The listing builds one solid part. Answer for the finished solid, in the listing's coordinates (mm). Face numbers are marked on the shaded views. A direction names the side the tool comes from. Round coordinates to 2 decimals unless told otherwise and drop trailing zeros. Write each loop counter-clockwise with the first axis right and the second up, starting at its lowest first coordinate (ties: lowest second). Pieces come first, ordered by that corner, then holes.
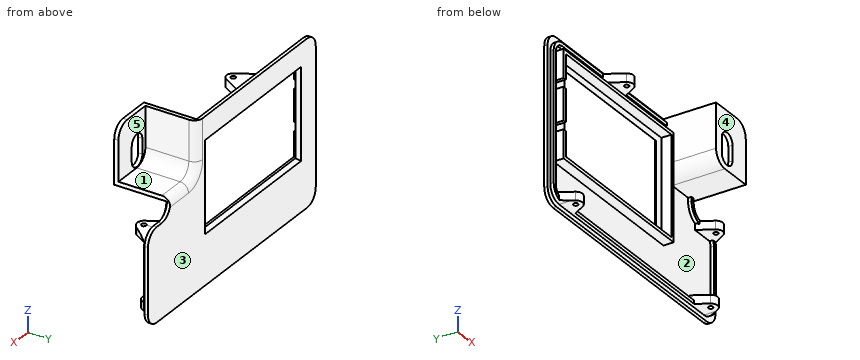
from build123d import *

# Parameters (mm, degrees)
BOSS_EXTRUDE1_DEPTH = 2
BOSS_EXTRUDE2_DEPTH = 2
SKETCH3_W           = 27.22
SKETCH3_H           = 33.28
BOSS_EXTRUDE3_DEPTH = 2.5
SKETCH4_W           = 31.75
SKETCH4_H           = 33.28
BOSS_EXTRUDE4_DEPTH = 2.5
SKETCH5_W           = 27.22
SKETCH5_H           = 34.25
BOSS_EXTRUDE5_DEPTH = 2.5
FILLET1_R           = 8
CUT_EXTRUDE1_REACH  = 98.066
FILLET3_R           = 8
FILLET6_R           = 5
SKETCH7_W           = 101
SKETCH7_H           = 62.8
SKETCH7_W_2         = 97
SKETCH7_H_2         = 58.8
BOSS_EXTRUDE6_DEPTH = 6
CUT_EXTRUDE2_REACH  = 98.896
SKETCH8_W           = 84
SKETCH8_H           = 50
CHAMFER1_SIZE       = 2
BOSS_EXTRUDE7_START = -2.5
SKETCH9_R           = 1.4
BOSS_EXTRUDE7_DEPTH = 5
BOSS_EXTRUDE8_START = 3.75
SKETCH10_R          = 1.4
BOSS_EXTRUDE8_DEPTH = 5
SKETCH11_R          = 1.4
BOSS_EXTRUDE9_DEPTH = 5
CUT_EXTRUDE3_DEPTH  = 97.22727472
SKETCH13_W          = 2
SKETCH13_H          = 5
CUT_EXTRUDE4_DEPTH  = 6


with BuildPart() as part:
    # Sketch1 → Boss-Extrude1 (new body)
    with BuildSketch(Plane(origin=(0, 0, 0), x_dir=(1, 0, 0), z_dir=(0, 1, 0))):
        with BuildLine():
            Line((-77, 40.5), (-77, -40.5))
            ThreePointArc((-77, -40.5), (-74.656854249, -46.156854249), (-69, -48.5))
            Line((-69, -48.5), (29.28, -48.5))
            Line((29.28, -48.5), (29.28, -46))
            Line((29.28, -46), (29.28, -14.25))
            Line((29.28, -14.25), (54, -14.25))
            Line((54, -14.25), (56.5, -14.25))
            ThreePointArc((56.5, -14.25), (58.843145751, -8.593145751), (64.5, -6.25))
            Line((64.5, -6.25), (69, -6.25))
            ThreePointArc((69, -6.25), (74.656854249, -3.906854249), (77, 1.75))
            Line((77, 1.75), (77, 40.5))
            ThreePointArc((77, 40.5), (74.656854249, 46.156854249), (69, 48.5))
            Line((69, 48.5), (-69, 48.5))
            ThreePointArc((-69, 48.5), (-74.656854249, 46.156854249), (-77, 40.5))
        make_face()
    extrude(amount=BOSS_EXTRUDE1_DEPTH)

    # Sketch2 → Boss-Extrude2 (add)
    with BuildSketch(Plane.XZ):
        with BuildLine():
            Line((54, 11.75), (54, 14.25))
            Line((54, 14.25), (52, 14.25))
            Line((52, 14.25), (52, 11.75))
            ThreePointArc((52, 11.75), (54.928932188, 4.678932188), (62, 1.75))
            Line((62, 1.75), (66.5, 1.75))
            ThreePointArc((66.5, 1.75), (70.742640687, -0.007359313), (72.5, -4.25))
            Line((72.5, -4.25), (72.5, -38))
            ThreePointArc((72.5, -38), (70.742640687, -42.242640687), (66.5, -44))
            Line((66.5, -44), (-66.5, -44))
            ThreePointArc((-66.5, -44), (-70.742640687, -42.242640687), (-72.5, -38))
            Line((-72.5, -38), (-72.5, 38))
            ThreePointArc((-72.5, 38), (-70.742640687, 42.242640687), (-66.5, 44))
            Line((-66.5, 44), (29.28, 44))
            Line((29.28, 44), (29.28, 46))
            Line((29.28, 46), (-66.5, 46))
            ThreePointArc((-66.5, 46), (-72.156854249, 43.656854249), (-74.5, 38))
            Line((-74.5, 38), (-74.5, -38))
            ThreePointArc((-74.5, -38), (-72.156854249, -43.656854249), (-66.5, -46))
            Line((-66.5, -46), (66.5, -46))
            ThreePointArc((66.5, -46), (72.156854249, -43.656854249), (74.5, -38))
            Line((74.5, -38), (74.5, -4.25))
            ThreePointArc((74.5, -4.25), (72.156854249, 1.406854249), (66.5, 3.75))
            Line((66.5, 3.75), (62, 3.75))
            ThreePointArc((62, 3.75), (56.343145751, 6.093145751), (54, 11.75))
        make_face()
    extrude(amount=BOSS_EXTRUDE2_DEPTH)

    # Sketch3 → Boss-Extrude3 (add)
    with BuildSketch(Plane.XY.offset(14.25)):
        with Locations((42.89, -14.64)):
            Rectangle(SKETCH3_W, SKETCH3_H)
    extrude(amount=BOSS_EXTRUDE3_DEPTH)

    # Sketch4 → Boss-Extrude4 (add)
    with BuildSketch(Plane(origin=(29.28, 0, 0), x_dir=(0, 0, -1), z_dir=(1, 0, 0))):
        with Locations((-32.625, -14.64)):
            Rectangle(SKETCH4_W, SKETCH4_H)
    extrude(amount=BOSS_EXTRUDE4_DEPTH)

    # Sketch5 → Boss-Extrude5 (add)
    with BuildSketch(Plane.XZ.offset(31.28)):
        with Locations((42.89, 31.375)):
            Rectangle(SKETCH5_W, SKETCH5_H)
    extrude(amount=-BOSS_EXTRUDE5_DEPTH)

    # Fillet1
    fillet1_edges = [part.edges().sort_by_distance(p)[0] for p in [
        (56.5, -30.03, 48.5),
    ]]
    fillet(fillet1_edges, radius=FILLET1_R)

    # Sketch6 → Cut-Extrude1 (cut, up to next)
    with BuildSketch(Plane(origin=(0, -28.78, 0), x_dir=(1, 0, 0), z_dir=(0, 1, 0)), mode=Mode.PRIVATE) as cut_extrude1_sk1:
        with BuildLine():
            Line((44.31, -22.12), (44.31, -31.12))
            ThreePointArc((44.31, -31.12), (39.43, -36), (34.55, -31.12))
            Line((34.55, -31.12), (34.55, -22.12))
            ThreePointArc((34.55, -22.12), (39.43, -17.24), (44.31, -22.12))
        make_face()
    cut_extrude1_tool1 = extrude(cut_extrude1_sk1.sketch, amount=-CUT_EXTRUDE1_REACH, mode=Mode.PRIVATE) & part.part
    add(cut_extrude1_tool1.solids().sort_by_distance((39.43, -28.78, 26.62))[0], mode=Mode.SUBTRACT)

    # Fillet3
    fillet3_edges = [part.edges().sort_by_distance(p)[0] for p in [
        (29.28, -15.64, 14.25),
        (31.78, -13.39, 16.75),
    ]]
    fillet(fillet3_edges, radius=FILLET3_R)

    # Fillet6
    fillet6_edges = [part.edges().sort_by_distance(p)[0] for p in [
        (31.78, 2, 36.625),
        (34.123145751, 2, 19.093145751),
        (48.14, 2, 16.75),
    ]]
    fillet(fillet6_edges, radius=FILLET6_R)

    # Sketch7 → Boss-Extrude6 (add)
    with BuildSketch(Plane.XZ):
        with Locations((-21.12, 7.52)):
            Rectangle(SKETCH7_W, SKETCH7_H)
        with Locations((-21.12, 7.52)):
            Rectangle(SKETCH7_W_2, SKETCH7_H_2, mode=Mode.SUBTRACT)
    extrude(amount=BOSS_EXTRUDE6_DEPTH)

    # Sketch8 → Cut-Extrude2 (cut, up to next)
    with BuildSketch(Plane(origin=(0, 2, 0), x_dir=(1, 0, 0), z_dir=(0, 1, 0)), mode=Mode.PRIVATE) as cut_extrude2_sk1:
        with Locations((-19.42, -7.92)):
            Rectangle(SKETCH8_W, SKETCH8_H)
    cut_extrude2_tool1 = extrude(cut_extrude2_sk1.sketch, amount=-CUT_EXTRUDE2_REACH, mode=Mode.PRIVATE) & part.part
    add(cut_extrude2_tool1.solids().sort_by_distance((-19.42, 2, 7.92))[0], mode=Mode.SUBTRACT)

    # Chamfer1
    chamfer1_edges = [part.edges().sort_by_distance(p)[0] for p in [
        (-19.42, 2, 32.92),
        (-61.42, 2, 7.92),
        (-19.42, 2, -17.08),
        (22.58, 2, 7.92),
    ]]
    chamfer(chamfer1_edges, length=CHAMFER1_SIZE - 0.0001)  # a hair under: the kernel refuses the full size

    # Sketch9 → Boss-Extrude7 (add)
    with BuildSketch(Plane.XY.offset(48.5).offset(BOSS_EXTRUDE7_START)):
        with BuildLine():
            Line((-23.324101615, -12), (-30.252304845, 0))
            Line((-30.252304845, 0), (-9.467695155, 0))
            Line((-9.467695155, 0), (-16.395898385, -12))
            ThreePointArc((-16.395898385, -12), (-19.86, -14), (-23.324101615, -12))
        make_face()
        with Locations(Location((-19.86, -10, 0), (0, 0, 180))):
            Circle(SKETCH9_R, mode=Mode.SUBTRACT)
    extrude(amount=-BOSS_EXTRUDE7_DEPTH)

    # Sketch10 → Boss-Extrude8 (add)
    with BuildSketch(Plane.XY.offset(BOSS_EXTRUDE8_START)):
        with BuildLine():
            Line((70.214101615, -9), (75.410254038, 0))
            Line((75.410254038, 0), (58.089745962, 0))
            Line((58.089745962, 0), (63.285898385, -9))
            ThreePointArc((63.285898385, -9), (66.75, -11), (70.214101615, -9))
        make_face()
        with Locations(Location((66.75, -7, 0), (0, 0, 180))):
            Circle(SKETCH10_R, mode=Mode.SUBTRACT)
    extrude(amount=-BOSS_EXTRUDE8_DEPTH)

    # Sketch11 → Boss-Extrude9 (add)
    # profile 1 of 2: a face of its own
    with BuildSketch(Plane(origin=(0, 0, -46), x_dir=(-1, 0, 0), z_dir=(0, 0, -1))):
        with BuildLine():
            Line((-65.464101615, -9), (-70.660254038, 0))
            Line((-70.660254038, 0), (-53.339745962, 0))
            Line((-53.339745962, 0), (-58.535898385, -9))
            ThreePointArc((-58.535898385, -9), (-62, -11), (-65.464101615, -9))
        make_face()
        with Locations((-62, -7)):
            Circle(SKETCH11_R, mode=Mode.SUBTRACT)
    # profile 2 of 2: a face of its own
    with BuildSketch(Plane(origin=(0, 0, -46), x_dir=(-1, 0, 0), z_dir=(0, 0, -1))):
        with BuildLine():
            Line((58.535898385, -9), (53.339745962, 0))
            Line((53.339745962, 0), (70.660254038, 0))
            Line((70.660254038, 0), (65.464101615, -9))
            ThreePointArc((65.464101615, -9), (62, -11), (58.535898385, -9))
        make_face()
        with Locations((62, -7)):
            Circle(SKETCH11_R, mode=Mode.SUBTRACT)
    extrude(amount=-BOSS_EXTRUDE9_DEPTH)

    # Sketch12 → Cut-Extrude3 (cut, through all)
    with BuildSketch(Plane.XZ):
        with BuildLine():
            Line((-66.5, -46), (66.5, -46))
            ThreePointArc((66.5, -46), (72.156854249, -43.656854249), (74.5, -38))
            Line((74.5, -38), (84.295668918, -38))
            Line((84.295668918, -38), (84.295668918, -62.929633478))
            Line((84.295668918, -62.929633478), (-82.125682446, -61.467965399))
            Line((-82.125682446, -61.467965399), (-82.125682446, -38))
            Line((-82.125682446, -38), (-74.5, -38))
            ThreePointArc((-74.5, -38), (-72.156854249, -43.656854249), (-66.5, -46))
        make_face()
        with BuildLine():
            Line((66.5, 3.75), (62, 3.75))
            ThreePointArc((62, 3.75), (56.343145751, 6.093145751), (54, 11.75))
            Line((54, 11.75), (84.295668918, 11.75))
            Line((84.295668918, 11.75), (84.295668918, -4.25))
            Line((84.295668918, -4.25), (74.5, -4.25))
            ThreePointArc((74.5, -4.25), (72.156854249, 1.406854249), (66.5, 3.75))
        make_face()
    extrude(amount=CUT_EXTRUDE3_DEPTH, mode=Mode.SUBTRACT)

    # Sketch13 → Cut-Extrude4 (cut)
    with BuildSketch(Plane.XZ.offset(6)):
        with Locations((-70.62, 19.72)):
            Rectangle(SKETCH13_W, SKETCH13_H)
        with Locations((-70.62, -4.68)):
            Rectangle(SKETCH13_W, SKETCH13_H)
    extrude(amount=-CUT_EXTRUDE4_DEPTH, mode=Mode.SUBTRACT)


solid = part.part
1. Straight lines are drawn through the part: line 1 along Z through (x, y) = (-7.5, -1.5); line 2 along Z through (x, y) = (-22.5, -1.5); line 3 along Y through (x, z) = (66.75, 0.2). For each, find the intervals that lie inside material, in ascending order.
Geometry says:
line 1: z = -46 to -44, -23.88 to -21.88, 36.92 to 38.92, 44 to 46
line 2: z = -46 to -44, -23.88 to -21.88, 36.92 to 38.92, 41 to 46
line 3: y = -11 to -8.4, -5.6 to 2
2. A tool of negligible diameter and unlimited length cuts with its end or side. For the marked faces 4 and 5, from which of +Z, -Z, +X, -X, +Y, -Y can it reach the whole face along a straight path? Write none if from no direction.
Geometry says:
face 4: +Z, -Z, +X, -X, -Y
face 5: +Z, +X, +Y
3. Given pin 1 (2 mm diameter, centred on x = 62, y = -3, fed in from +Z); pin 2 (6.5 mm diameter, centred on x = -8.5, y = -3.5, fed in from -Z); pin 3 (9 mm diameter, centred on x = 8.5, y = -4, fed in from -Z); pin 4 (6 mm diameter, centred on x = -41.5, z = 29.5, fed in from +Y), each flat-ended and moving along its own axis, determine where each tip first touches the part or whether it passes through.
Geometry says:
pin 1: stops at z = 3.75
pin 2: stops at z = -46
pin 3: stops at z = -48.5
pin 4: passes through
4. Section C-C on z = -27 is taken. Determine the outline of the cut face in (x, y), plus the area to 3 significant figures.
Geometry says:
outline: (-77, 0) - (-74.5, 0) - (-74.5, -2) - (-72.5, -2) - (-72.5, 0) - (72.5, 0) - (72.5, -2) - (74.5, -2) - (74.5, 0) - (77, 0) - (77, 2) - (-77, 2) - close
area: 316 mm2
5. Section D-D on y = -27 is taken. Determine the outline of the cut face in (x, z), plus the area to 3 significant figures.
Geometry says:
outline: (29.28, 22.25) arc R8 ccw to (37.28, 14.25) - (56.5, 14.25) - (56.5, 16.75) - (39.78, 16.75) arc R8 cw to (31.78, 24.75) - (31.78, 48.5) - (29.28, 48.5) - close
area: 147 mm2
6. For a pull along Z with two mould halves and no side action, classify the marked faces 1, 2 and 3 as released by +Z, released by -Z, zero draft, split by the parting line, or undercut.
Geometry says:
face 1: released by +Z
face 2: undercut
face 3: zero draft
